```python
from build123d import *

# Parameters (mm, degrees)
F0_W     = 165.1
F0_H     = 101.6
F1_DEPTH = 12.7
F2_W     = 82.296
F2_H     = 101.6
F3_DEPTH = 25.4
F5_D     = 6.35
F5_DEPTH = 19.05
F5_TIP   = 1.9077324654


with BuildPart() as f1:
    # F0 (on Top) → F1 (new body)
    with BuildSketch(Plane.XY):
        Rectangle(F0_W, F0_H)
        with BuildLine():
            ThreePointArc((-73.152, -43.688), (-78.74, -38.1), (-73.152, -32.512))
            Line((-73.152, -32.512), (-50.8, -32.512))
            ThreePointArc((-50.8, -32.512), (-45.212, -38.1), (-50.8, -43.688))
            Line((-50.8, -43.688), (-73.152, -43.688))
        make_face(mode=Mode.SUBTRACT)
        with BuildLine():
            ThreePointArc((73.152, -32.512), (78.74, -38.1), (73.152, -43.688))
            Line((73.152, -43.688), (50.8, -43.688))
            ThreePointArc((50.8, -43.688), (45.212, -38.1), (50.8, -32.512))
            Line((50.8, -32.512), (73.152, -32.512))
        make_face(mode=Mode.SUBTRACT)
        with BuildLine():
            Line((-50.8, 32.512), (-73.152, 32.512))
            ThreePointArc((-73.152, 32.512), (-78.74, 38.1), (-73.152, 43.688))
            Line((-73.152, 43.688), (-50.8, 43.688))
            ThreePointArc((-50.8, 43.688), (-45.212, 38.1), (-50.8, 32.512))
        make_face(mode=Mode.SUBTRACT)
        with BuildLine():
            ThreePointArc((50.8, 32.512), (45.212, 38.1), (50.8, 43.688))
            Line((50.8, 43.688), (73.152, 43.688))
            ThreePointArc((73.152, 43.688), (78.74, 38.1), (73.152, 32.512))
            Line((73.152, 32.512), (50.8, 32.512))
        make_face(mode=Mode.SUBTRACT)
    extrude(amount=F1_DEPTH)

    # F2 (on face) → F3 (join)
    with BuildSketch(Plane.XY.offset(12.7)):
        Rectangle(F2_W, F2_H)
    extrude(amount=F3_DEPTH)

    # F5
    with Locations(Plane.XY.offset(38.1)):
        with Locations((-31.75, 17.526), (-31.75, -17.526), (31.75, -17.526), (31.75, 17.526)):
            Hole(F5_D / 2, depth=F5_DEPTH)
            with Locations((0, 0, -(F5_DEPTH + F5_TIP / 2))):  # 118° drill point
                Cone(0, F5_D / 2, F5_TIP, mode=Mode.SUBTRACT)


solid = f1.part
```
Source: CAD feature listing. Evaluate the final solid. Frame: model axes, mm. A direction names the side the tool comes from. Round coordinates to 2 decimals unless told otherwise and drop trailing zeros. Loops run counter-clockwise (first coordinate to the right, second up) from the corner with the lowest first, then second, coordinate; pieces in that order, holes last.
(1) Material intervals for probe 1 along Y at (x, z) = (-72.5, 4); probe 2 along Y at (x, z) = (-31.75, 31.5); probe 3 along X at (y, z) = (6, 27.5), sorted ascending.
From the geometry:
probe 1: y = -50.8 to -43.69, -32.51 to 32.51, 43.69 to 50.8
probe 2: y = -50.8 to -20.7, -14.35 to 14.35, 20.7 to 50.8
probe 3: x = -41.15 to 41.15
(2) Section query D-D (z = 35.5). Output: boundary loops of the cut face in (x, y) (3 decimals).
From the geometry:
outline: (-41.148, -50.8) - (41.148, -50.8) - (41.148, 50.8) - (-41.148, 50.8) - close; hole circle Ø6.35 at (-31.75, -17.526); hole circle Ø6.35 at (-31.75, 17.526); hole circle Ø6.35 at (31.75, -17.526); hole circle Ø6.35 at (31.75, 17.526)
(3) Access query for faces 1 (the flat face through (-1, 50.8, 15)), 2 (the flat face through (62, 1, 12.7)), 3 (the cylindrical face through (-31.062, -20.625, 28.442)), 4 (the flat face through (62, -43.688, 6)), 5 (the flat face through (-82.55, -1, 6)). Directions: +Z, -Z, +X, -X, +Y, -Y. A direction counts if a zero-diameter tool reaches every point of the face in a straight line with its end or side. Return the directions, or none.
From the geometry:
face 1: +Z, -Z, +X, -X, +Y
face 2: +Z, +X, +Y, -Y
face 3: +Z
face 4: +Z, -Z
face 5: +Z, -Z, -X, +Y, -Y
(4) Section query B-B (y = -38.1). Output: boundary loops of the cut face in (x, z).
From the geometry:
outline: (-82.55, 0) - (-78.74, 0) - (-78.74, 12.7) - (-82.55, 12.7) - close; (-45.21, 0) - (45.21, 0) - (45.21, 12.7) - (41.15, 12.7) - (41.15, 38.1) - (-41.15, 38.1) - (-41.15, 12.7) - (-45.21, 12.7) - close; (78.74, 0) - (82.55, 0) - (82.55, 12.7) - (78.74, 12.7) - close
(5) Section query C-C (z = 5). Output: boundary loops of the cut face in (x, y), and give its area (3 significant figures).
From the geometry:
outline: (-82.55, -50.8) - (82.55, -50.8) - (82.55, 50.8) - (-82.55, 50.8) - close; hole (-73.15, -43.69) - (-50.8, -43.69) arc R5.59 ccw to (-50.8, -32.51) - (-73.15, -32.51) arc R5.59 ccw to start; hole (-73.15, 32.51) - (-50.8, 32.51) arc R5.59 ccw to (-50.8, 43.69) - (-73.15, 43.69) arc R5.59 ccw to start; hole (50.8, -43.69) - (73.15, -43.69) arc R5.59 ccw to (73.15, -32.51) - (50.8, -32.51) arc R5.59 ccw to start; hole (50.8, 32.51) - (73.15, 32.51) arc R5.59 ccw to (73.15, 43.69) - (50.8, 43.69) arc R5.59 ccw to start
area: 15,400 mm2
(6) Contact query for flat-ended pins moving along their axis: pin 1 Ø7.5 at (y, z) = (-2, 19.5) entering from +X; pin 2 Ø10 at (y, z) = (23.5, 26) entering from -X; pin 3 Ø20.5 at (x, y) = (70.5, 25) entering from +Z; pin 4 Ø8 at (x, z) = (-63, 17) entering from +Y. Output: stop coordinate, or through.
From the geometry:
pin 1: stops at x = 41.15
pin 2: stops at x = -41.15
pin 3: stops at z = 12.7
pin 4: passes through
(7) Pull-direction query (X, two-part tool) for faces 6 (the flat face through (-41.148, -1, 25)), 7 (the flat face through (-1, 1, 38.1)), 8 (the cylindrical face through (78.74, 38.22, 6.26)); classes: +X half, -X half, draft (parallel to the pull), parting line (faces both ways), or undercut.
From the geometry:
face 6: -X half
face 7: draft
face 8: undercut
(8) Section query A-A (x = -54.5). Output: boundary loops of the cut face in (y, z), and give its area (3 significant figures).
From the geometry:
outline: (-50.8, 0) - (-43.69, 0) - (-43.69, 12.7) - (-50.8, 12.7) - close; (-32.51, 0) - (32.51, 0) - (32.51, 12.7) - (-32.51, 12.7) - close; (43.69, 0) - (50.8, 0) - (50.8, 12.7) - (43.69, 12.7) - close
area: 1,010 mm2
